Model file for the job. Use its own axes, mm. A direction names the side the tool comes from. Give positions to 0.01 mm unless a question says otherwise; leave off trailing zeros. Loops run counter-clockwise (first coordinate to the right, second up) from the corner with the lowest first, then second, coordinate; pieces in that order, holes last. Notation, with made-up numbers: M 20,40 L 30,40 A14 ccw 30,60 Z; hole C -35,28 d4. An arc over 180 degrees is marked long. Use CSV: the item, a comma, the result in double quotes. Start each with the question number.
(1) Slice it at C-C on y = 50. List the corners of the cut face in (x, z) (3 decimals).
(2) Two-plate mould, pull along X, no slides. Class faces 1 (the face through (0, 90, 8.306)), 2 (the face through (-8.306, 88, 0)), 3 (the face through (0, 92, 9.525)), 4 (the face through (9.525, 88, 0)): pulls with the +X half, pulls with the -X half, needs draft (parallel to the pull), parting line crosses it, or undercut.
(3) Slice it at D-D on z = -6. List the corners of the cut face in (x, y) (3 decimals).
(4) Wall check: line 1 along Y through (x, z) = (9.1, 0); line 2 along X through (y, z) = (37.5, 7.25) (3 decimals); line 3 along Z through (x, y) = (-8.65, 50) (3 decimals). Give the ranges that are in metal, low to high. Write a range as from..to.
(5) Slice it at B-B on y = 21.5. List the corners of the cut face in (x, z) (3 decimals), and give its area (3 significant figures).
(6) Slice it at A-A on x = -0.25. List the corners of the cut face in (y, z) (3 decimals).
(7) Tool access for faces 5 (the face through (0, 90, -8.306)), 6 (the face through (8.907, 53.549, -1.846)): list every direction of +Z, -Z, +X, -X, +Y, -Y with a clear straight run to the whole face (end or side of a thin tool).
Autodesk Inventor part; units mm, degrees
ref_plane "YZ Plane" through (0, 0, 0) normal (1, 0, 0) x (0, 1, 0)
ref_plane "XZ Plane" through (0, 0, 0) normal (0, 1, 0) x (-1, 0, 0)
ref_plane "XY Plane" through (0, 0, 0) normal (0, 0, 1) x (1, 0, 0)
sketch "Sketch4" plane through (0, 0, 0) normal (0, 1, 0) x (-1, 0, 0)
  line L0 (-9.525, -9.525) -> (9.525, -9.525)
  line L1 (9.525, -9.525) -> (9.525, 9.525)
  line L2 (9.525, 9.525) -> (-9.525, 9.525)
  line L3 (-9.525, 9.525) -> (-9.525, -9.525)
  line L4 (0, -13.335) -> (0, 13.335) construction
  line L5 (13.335, 0) -> (-13.335, 0) construction
  line L6 (-8.3058, 8.3058) -> (8.3058, 8.3058)
  line L7 (8.3058, 8.3058) -> (8.3058, -8.3058)
  line L8 (8.3058, -8.3058) -> (-8.3058, -8.3058)
  line L9 (-8.3058, -8.3058) -> (-8.3058, 8.3058)
  point P0 (0, 0)
  dimension "d44" = 19.05
  dimension "d45" = 1.2192
extrude "Extrusion2" add sketch "Sketch4" along normal blind 177.8
sketch "Sketch5" plane through (0, 0, 0) normal (1, 0, 0) x (0, 1, 0)
  line L0 (0, 115.5) -> (0, -115.5) construction
  line L1 (-33, 0) -> (198, 0) construction
  line L2 (165, 0) -> (135, 0)
  point P0 (0, 0)
  point P1 (50, 0)
  point P2 (15, 0)
  point P3 (150, 0)
  dimension "d48" = 15
  dimension "d49" = 50
  dimension "d50" = 30
  dimension "d51" = 135
  dimension "d59" = 150
hole "Hole2" at (0, 50, 0) at (0, 15, 0) at (0, 165, 0) at (0, 135, 0) direction (-1, 0, 0) diameter 8 end through all both
fillet "Fillet2" radius 8 2 edges at (0, 0, -9.525) (0, 0, 9.525)
properties part number "Pedalbox_V2_Brake_Extrusion"
Reply:
1,outline,"M -9.525,-9.525 L 9.525,-9.525 L 9.525,-4 L 8.306,-4 L 8.306,-8.306 L -8.306,-8.306 L -8.306,-4 L -9.525,-4 Z; M -9.525,4 L -8.306,4 L -8.306,8.306 L 8.306,8.306 L 8.306,4 L 9.525,4 L 9.525,9.525 L -9.525,9.525 Z"
2,face 1,"undercut"
2,face 2,"undercut"
2,face 3,"needs draft"
2,face 4,"pulls with the +X half"
3,outline,"M -9.525,1.369 L -8.306,1.369 L -8.306,177.8 L -9.525,177.8 Z; M 8.306,1.369 L 9.525,1.369 L 9.525,177.8 L 8.306,177.8 Z"
4,line 1,"y = 0..11, 19..46, 54..131, 139..161, 169..177.8"
4,line 2,"x = -9.525..-8.306, 8.306..9.525"
4,line 3,"z = -9.525..-4, 4..9.525"
5,outline,"M -9.525,-9.525 L 9.525,-9.525 L 9.525,9.525 L -9.525,9.525 Z; hole M -8.306,-8.306 L 8.306,-8.306 L 8.306,8.306 L -8.306,8.306 Z"
5,area,"87.0 mm^2"
6,outline,"M 3.755,-8.306 A8 ccw 8,-9.525 L 177.8,-9.525 L 177.8,-8.306 Z; M 3.755,8.306 L 177.8,8.306 L 177.8,9.525 L 8,9.525 A8 ccw Z"
7,face 5,"+Y, -Y"
7,face 6,"+X, -X"
